from build123d import *

# Parameters (mm, degrees)
SKETCH1_R               = 20
BOSS_EXTRUDE1_DEPTH     = 6
SKETCH2_R               = 2
CUT_EXTRUDE1_DEPTH      = 7
CUT_EXTRUDE1_DEPTH_BACK = 29.91366459
SKETCH3_R               = 15
CUT_EXTRUDE2_DEPTH      = 6
SKETCH4_R               = 30
SKETCH4_R_2             = 15
BOSS_EXTRUDE2_DEPTH     = 5
SKETCH6_R               = 2
CUT_EXTRUDE3_DEPTH      = 7
CUT_EXTRUDE4_DEPTH      = 4
SKETCH8_R               = 2.5
CUT_EXTRUDE5_DEPTH      = 4
SKETCH9_R               = 32.5
SKETCH9_R_2             = 30
BOSS_EXTRUDE3_DEPTH     = 1


with BuildPart() as part:
    # Sketch1 → Boss-Extrude1 (new body)
    with BuildSketch(Plane.XY):
        Circle(SKETCH1_R)
    extrude(amount=BOSS_EXTRUDE1_DEPTH)

    # Sketch2 → Cut-Extrude1 (cut, two sides)
    with BuildSketch(Plane.XY.offset(6)) as cut_extrude1_sk:
        with Locations((0, 17.5)):
            Circle(SKETCH2_R)
        with Locations((12.374368671, 12.374368671)):
            Circle(SKETCH2_R)
        with Locations((17.5, 0)):
            Circle(SKETCH2_R)
        with Locations((12.374368671, -12.374368671)):
            Circle(SKETCH2_R)
        with Locations((0, -17.5)):
            Circle(SKETCH2_R)
        with Locations((-12.374368671, -12.374368671)):
            Circle(SKETCH2_R)
        with Locations((-17.5, 0)):
            Circle(SKETCH2_R)
        with Locations((-12.374368671, 12.374368671)):
            Circle(SKETCH2_R)
    extrude(amount=CUT_EXTRUDE1_DEPTH, mode=Mode.SUBTRACT)
    extrude(cut_extrude1_sk.sketch, amount=-CUT_EXTRUDE1_DEPTH_BACK, mode=Mode.SUBTRACT)

    # Sketch3 → Cut-Extrude2 (cut)
    with BuildSketch(Plane(origin=(0, 0, 0), x_dir=(-1, 0, 0), z_dir=(0, 0, -1))):
        Circle(SKETCH3_R)
    extrude(amount=-CUT_EXTRUDE2_DEPTH, mode=Mode.SUBTRACT)

    # Sketch4 → Boss-Extrude2 (add)
    with BuildSketch(Plane.XY.offset(6)):
        Circle(SKETCH4_R)
        with Locations(Location((0, 0, 0), (0, 0, 180))):
            Circle(SKETCH4_R_2, mode=Mode.SUBTRACT)
    extrude(amount=BOSS_EXTRUDE2_DEPTH)

    # Sketch6 → Cut-Extrude3 (cut)
    with BuildSketch(Plane(origin=(0, 0, 6), x_dir=(-1, 0, 0), z_dir=(0, 0, -1))):
        with Locations(Location((0, 17.5, 0), (0, 0, 180))):
            Circle(SKETCH6_R)
        with Locations(Location((12.374368671, 12.374368671, 0), (0, 0, 180))):
            Circle(SKETCH6_R)
        with Locations(Location((17.5, 0, 0), (0, 0, 180))):
            Circle(SKETCH6_R)
        with Locations(Location((12.374368671, -12.374368671, 0), (0, 0, 180))):
            Circle(SKETCH6_R)
        with Locations(Location((0, -17.5, 0), (0, 0, 180))):
            Circle(SKETCH6_R)
        with Locations(Location((-12.374368671, -12.374368671, 0), (0, 0, 180))):
            Circle(SKETCH6_R)
        with Locations(Location((-17.5, 0, 0), (0, 0, 180))):
            Circle(SKETCH6_R)
        with Locations(Location((-12.374368671, 12.374368671, 0), (0, 0, 180))):
            Circle(SKETCH6_R)
    extrude(amount=-CUT_EXTRUDE3_DEPTH, mode=Mode.SUBTRACT)

    # Sketch7 → Cut-Extrude4 (cut)
    with BuildSketch(Plane(origin=(0, 0, 6), x_dir=(-1, 0, 0), z_dir=(0, 0, -1))):
        Polygon((23.960036171, 8.5), (26.269437248, 12.5), (23.960036171, 16.5), (19.341234018, 16.5), (17.031832941, 12.5), (19.341234018, 8.5), align=None)
        Polygon((4.618802154, 25), (2.309401077, 29), (-2.309401077, 29), (-4.618802154, 25), (-2.309401077, 21), (2.309401077, 21), align=None)
        Polygon((19.341234018, -16.5), (23.960036171, -16.5), (26.269437248, -12.5), (23.960036171, -8.5), (19.341234018, -8.5), (17.031832941, -12.5), align=None)
        Polygon((-4.618802154, -25), (-2.309401077, -29), (2.309401077, -29), (4.618802154, -25), (2.309401077, -21), (-2.309401077, -21), align=None)
        Polygon((-23.960036171, -8.5), (-26.269437248, -12.5), (-23.960036171, -16.5), (-19.341234018, -16.5), (-17.031832941, -12.5), (-19.341234018, -8.5), align=None)
        Polygon((-19.341234018, 16.5), (-23.960036171, 16.5), (-26.269437248, 12.5), (-23.960036171, 8.5), (-19.341234018, 8.5), (-17.031832941, 12.5), align=None)
    extrude(amount=-CUT_EXTRUDE4_DEPTH, mode=Mode.SUBTRACT)

    # Sketch8 → Cut-Extrude5 (cut)
    with BuildSketch(Plane(origin=(0, 0, 10), x_dir=(-1, 0, 0), z_dir=(0, 0, -1))):
        with Locations((0, 25)):
            Circle(SKETCH8_R)
        with Locations((21.650635095, 12.5)):
            Circle(SKETCH8_R)
        with Locations((21.650635095, -12.5)):
            Circle(SKETCH8_R)
        with Locations((0, -25)):
            Circle(SKETCH8_R)
        with Locations((-21.650635095, -12.5)):
            Circle(SKETCH8_R)
        with Locations((-21.650635095, 12.5)):
            Circle(SKETCH8_R)
    extrude(amount=-CUT_EXTRUDE5_DEPTH, mode=Mode.SUBTRACT)

    # Sketch9 → Boss-Extrude3 (add)
    with BuildSketch(Plane(origin=(0, 0, 6), x_dir=(-1, 0, 0), z_dir=(0, 0, -1))):
        Circle(SKETCH9_R)
        Circle(SKETCH9_R_2, mode=Mode.SUBTRACT)
    extrude(amount=-BOSS_EXTRUDE3_DEPTH)


solid = part.part
Model file for the job. Use its own axes, mm. A direction names the side the tool comes from. Coordinates: 2 decimals unless noted, no trailing zeros. Write each loop counter-clockwise with the first axis right and the second up, starting at its lowest first coordinate (ties: lowest second). Pieces come first, ordered by that corner, then holes. Notation, with made-up numbers: (-1.5, -35.75) - (2.5, -35.75) arc R17 cw to (2.5, -4.75) - close; hole circle Ø9 at (89, 10.25). An arc over 180 degrees is marked (long way). Write each question's results on one line, items separated by ' | '. Start each with the question number.
1) Cut at A-A (x = 8.5). Write the cut outline in (y, z), then the cut area to 3 significant figures.
2) Cut at C-C (z = 4.5). Count the separate pieces of the cut face and the enclosed holes in it, then the cut area to 3 significant figures.
3) Flat gauge pins, fed straight in: P1, Ø4.5, axis at x = -21, z = 7.5, coming from the -Y side; P2, Ø1, axis at y = -25.5, z = 5, coming from the +X side; P3, Ø9, axis at x = -23, y = 13, coming from the -Z side; P4, Ø2, axis at x = 20.5, z = 7.5, coming from the +Y side. Where does each tip first touch, or does it go through?
4) 3-axis set-ups, long thin cutter, end or side, ignore diameter. For faces 1 (the face through (-13.962, 13.591, 5.423)), 2 (the face through (0, 21, 8)): which of +Z, -Z, +X, -X, +Y, -Y reach the whole face in a straight line?
5) Mould opens along X. For faces 3 (the face through (-9, -29, 7)), 4 (the face through (-23.96, -13.46, 10.49)) say: pulls with the +X half, pulls with the -X half, needs draft (parallel to the pull), parting line crosses it, or undercut.
6) Probe line 1 along Y through (x, z) = (0, 2.5); line 2 along Y through (x, z) = (-13, 9.75); line 3 along Y through (x, z) = (0, 10.75). List the from-to ranges inside material, lowest first. Write a range as from..to.
7) Cut at B-B (y = -4.5). Write the cut outline in (x, z), then the cut area to 3 significant figures.
Returned:
1) outline: (-31.37, 6) - (-18.1, 6) - (-18.1, 0) - (-12.36, 0) - (-12.36, 11) - (-28.77, 11) - (-28.77, 7) - (-31.37, 7) - close; (12.36, 0) - (18.1, 0) - (18.1, 6) - (31.37, 6) - (31.37, 7) - (28.77, 7) - (28.77, 11) - (12.36, 11) - close | area: 238 mm^2
2) separate pieces: 1 | enclosed holes: 9 | area: 449 mm^2
3) P1: y = -26.51 | P2: through | P3: z = 6 | P4: y = 25.9
4) face 1: +Z, -Z | face 2: -Z
5) face 3: needs draft | face 4: undercut
6) line 1: -20..-19.5, -15.5..-15, 15..15.5, 19.5..20 | line 2: -27.04..-14.27, -10.47..-7.48, 7.48..10.47, 14.27..27.04 | line 3: -30..-27.5, -22.5..-19.5, -15.5..-15, 15..15.5, 19.5..22.5, 27.5..30
7) outline: (-32.19, 6) - (-19.49, 6) - (-19.49, 0) - (-14.31, 0) - (-14.31, 11) - (-29.66, 11) - (-29.66, 7) - (-32.19, 7) - close; (14.31, 0) - (19.49, 0) - (19.49, 6) - (32.19, 6) - (32.19, 7) - (29.66, 7) - (29.66, 11) - (14.31, 11) - close | area: 221 mm^2
